The listing builds one solid part. Answer for the finished solid, in the listing's coordinates (mm). A direction names the side the tool comes from. Coordinates: 2 decimals unless noted, no trailing zeros. Order: outer loops, then holes, each group sorted by start corner. A loop starts at its lowest first (then second) coordinate and runs counter-clockwise, first axis right, second up. Notation, with made-up numbers: (81.5, -1.5) -> (101.5, -1.5) arc R16 cw to (101.5, 21.5) -> close; hole circle Ø8 at (84, 77). An arc over 180 degrees is marked (long way). Write item = value, one per line. Start each with the question number.
```python
from build123d import *

# Parameters (mm, degrees)
BOSS_EXTRUDE1_DEPTH = 2133.6
CUT_EXTRUDE2_DEPTH  = 613.218203925
SHELL1_T            = -7.9375
SKETCH14_R          = 38.1
SKETCH14_R_2        = 15.875
BOSS_EXTRUDE2_DEPTH = 12.7


with BuildPart() as part:
    # Sketch1 → Boss-Extrude1 (new body)
    with BuildSketch(Plane.XY):
        Polygon((0, 0), (508, 0), (660.4, 406.4), (-152.4, 406.4), align=None)
    extrude(amount=BOSS_EXTRUDE1_DEPTH)

    # Sketch13 → Cut-Extrude2 (cut, symmetric, along a direction that is not the sketch's normal)
    with BuildSketch(Plane(origin=(254, 0, 0), x_dir=(0, 0, -1), z_dir=(1, 0, 0))):
        Polygon((-2133.6, 0), (-3174.648587482, 0), (-3174.648587482, 406.4), (-2133.6, 406.4), (-1676.4, 0), align=None)
    cut_extrude2 = extrude(amount=CUT_EXTRUDE2_DEPTH, dir=(0.664363839, 0, 0.747409319), both=True, mode=Mode.SUBTRACT)

    # Mirror1: Cut-Extrude2 across plane
    add(cut_extrude2.mirror(Plane(origin=(254, 0, 0), x_dir=(0, 0, 1), z_dir=(1, 0, 0))), mode=Mode.SUBTRACT)

    # Shell1
    shell1_openings = [part.faces().sort_by_distance(p)[0] for p in [
        (254, 406.4, 1097.28),
    ]]
    offset(amount=SHELL1_T, openings=shell1_openings, kind=Kind.INTERSECTION)

    # Sketch14 → Boss-Extrude2 (add)
    with BuildSketch(Plane(origin=(437.937750167, -164.226656313, 0), x_dir=(0, 0, 1), z_dir=(-0.936329178, 0.351123442, 0))):
        with Locations((58.7375, 380.829536089)):
            Circle(SKETCH14_R)
        with Locations((58.7375, 380.829536089)):
            Circle(SKETCH14_R_2, mode=Mode.SUBTRACT)
        with Locations((719.1375, 380.829536089)):
            Circle(SKETCH14_R)
        with Locations((719.1375, 380.829536089)):
            Circle(SKETCH14_R_2, mode=Mode.SUBTRACT)
        with Locations((1430.3375, 380.829536089)):
            Circle(SKETCH14_R)
        with Locations((1430.3375, 380.829536089)):
            Circle(SKETCH14_R_2, mode=Mode.SUBTRACT)
    boss_extrude2 = extrude(amount=BOSS_EXTRUDE2_DEPTH)

    # Mirror2: Boss-Extrude2 across plane
    add(boss_extrude2.mirror(Plane(origin=(254, 0, 0), x_dir=(0, 0, 1), z_dir=(1, 0, 0))))


solid = part.part
```
Item 1: Section D-D, the plane y = 272.5 is taken. Give the vertices of the cut face in (x, z).
Item 2: Consider probe 1 along Z at (x, y) = (166, 121.5); probe 2 along Y at (x, z) = (253, 276); probe 3 along Z at (x, y) = (562.5, 364.5). Determine where each line is inside the solid, lowest interval first.
Item 3: Section A-A, the plane z = 610 is taken. Give the vertices of the cut face in (x, y).
Item 4: Which of the six approach directions +Z, -Z, +X, -X, +Y, -Y give full straight-line access (tool end or side, diameter ignored) to faces 4 (the cylindrical face through (-44.73, 159.73, 50.48)), 5 (the flat face through (559.95, 197.31, 735.54))?
Item 5: Section C-C, the plane x = 216 is taken. Give the vertices of the cut face in (y, z).
Item 6: Section B-B, the plane y = 56.5 is taken. Give the vertices of the cut face in (x, z), then the cut area to 3 significant figures.
Item 7: For a pull along Y with two mould halves and no side action, classify faces 1 (the flat face through (559.95, 197.31, 1446.74)), 2 (the flat face through (250, 0, 826)), 3 (the cylindrical face through (560.67, 180.89, 754.332)) as pulls with the +Y half, pulls with the -Y half, needs draft (parallel to the pull), parting line crosses it, or undercut.
Item 8: Each of these flat-tipped pins is pushed along its axis until it touches: pin 1 (12 mm diameter, centred on y = 196, z = 1207.5, fed in from -X); pin 2 (8 mm diameter, centred on x = 372, z = 586, fed in from +Y); pin 3 (4 mm diameter, centred on x = 67.5, y = 105, fed in from +Z). Where does it stop, or does it pass through?
A:
q1.outline = (-102.19, 0) -> (610.19, 0) -> (610.19, 1582.25) -> (254, 1982.96) -> (-102.19, 1582.25) -> close; hole (-93.71, 7.94) -> (601.71, 7.94) -> (601.71, 1576.87) -> (254, 1968.05) -> (-93.71, 1576.87) -> close
q2.probe_1 = 0 to 7.94, 1699.17 to 1714.09
q2.probe_2 = 0 to 7.94
q2.probe_3 = 0 to 7.94, 1724.48 to 1739.4
q3.outline = (-152.4, 406.4) -> (0, 0) -> (508, 0) -> (660.4, 406.4) -> (651.92, 406.4) -> (502.5, 7.94) -> (5.5, 7.94) -> (-143.92, 406.4) -> close
q4.face_4 = none
q4.face_5 = +Y
q5.outline = (0, 0) -> (406.4, 0) -> (406.4, 7.94) -> (7.94, 7.94) -> (7.94, 1627.66) -> (406.4, 2075.93) -> (406.4, 2090.85) -> (0, 1633.65) -> close
q6.outline = (-21.19, 0) -> (529.19, 0) -> (529.19, 1430.38) -> (254, 1739.96) -> (-21.19, 1430.38) -> close; hole (-12.71, 7.94) -> (520.71, 7.94) -> (520.71, 1425) -> (254, 1725.05) -> (-12.71, 1425) -> close
q6.area = 36,500 mm^2
q7.face_1 = pulls with the +Y half
q7.face_2 = pulls with the -Y half
q7.face_3 = undercut
q8.pin_1 = -75.75
q8.pin_2 = 7.94
q8.pin_3 = 1587.89
